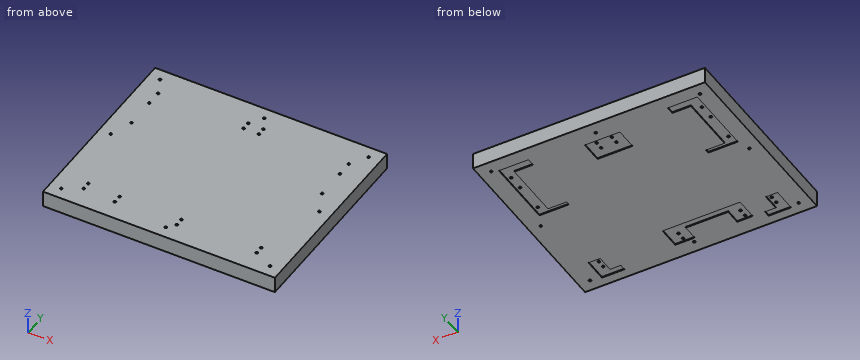
```python
from build123d import *

# Parameters (mm, degrees)
SKIZZE1_W                       = 300
SKIZZE1_H                       = 250
SKIZZE1_R                       = 1.6
AUFSATZ_LINEAR_AUSTRAGEN5_DEPTH = 21
SKIZZE2_R                       = 1.6
SKIZZE2_R_2                     = 1.5
SCHNITT_LINEAR_AUSTRAGEN2_DEPTH = 21
SKIZZE4_W                       = 45.307875895
SKIZZE4_H                       = 28.066825776
SCHNITT_LINEAR_AUSTRAGEN4_DEPTH = 1


with BuildPart() as part:
    # Skizze1 → Aufsatz-Linear austragen5 (new body)
    with BuildSketch(Plane.XY):
        with Locations((150, 125)):
            Rectangle(SKIZZE1_W, SKIZZE1_H)
        with Locations(Location((15, 15, 0), (0, 0, 180))):
            Circle(SKIZZE1_R, mode=Mode.SUBTRACT)
        with Locations(Location((285, 15, 0), (0, 0, 180))):
            Circle(SKIZZE1_R, mode=Mode.SUBTRACT)
        with Locations(Location((285, 235, 0), (0, 0, 180))):
            Circle(SKIZZE1_R, mode=Mode.SUBTRACT)
        with Locations(Location((15, 235, 0), (0, 0, 180))):
            Circle(SKIZZE1_R, mode=Mode.SUBTRACT)
        with Locations(Location((150, 15, 0), (0, 0, 180))):
            Circle(SKIZZE1_R, mode=Mode.SUBTRACT)
        with Locations(Location((285, 125, 0), (0, 0, 180))):
            Circle(SKIZZE1_R, mode=Mode.SUBTRACT)
        with Locations(Location((15, 125, 0), (0, 0, 180))):
            Circle(SKIZZE1_R, mode=Mode.SUBTRACT)
        with Locations(Location((150, 235, 0), (0, 0, 180))):
            Circle(SKIZZE1_R, mode=Mode.SUBTRACT)
    extrude(amount=AUFSATZ_LINEAR_AUSTRAGEN5_DEPTH)

    # Skizze2 → Schnitt-Linear austragen2 (cut)
    with BuildSketch(Plane.XY):
        with Locations(Location((158.603155074, 25.118294, 0), (0, 0, 180))):
            Circle(SKIZZE2_R)
        with Locations(Location((158.603155074, 35.36547744, 0), (0, 0, 180))):
            Circle(SKIZZE2_R)
        with Locations(Location((260.44562916, 27.513648646, 0), (0, 0, 180))):
            Circle(SKIZZE2_R)
        with Locations(Location((260.44562916, 37.512496181, 0), (0, 0, 180))):
            Circle(SKIZZE2_R)
        with Locations(Location((271.872836796, 153.81431076, 0), (0, 0, 180))):
            Circle(SKIZZE2_R)
        with Locations(Location((271.872850829, 193.508875377, 0), (0, 0, 180))):
            Circle(SKIZZE2_R)
        with Locations(Location((271.872850829, 213.356130747, 0), (0, 0, 180))):
            Circle(SKIZZE2_R)
        with Locations(Location((158.603451148, 218.134079373, 0), (0, 0, 180))):
            Circle(SKIZZE2_R)
        with Locations(Location((138.798289388, 208.167325209, 0), (0, 0, 180))):
            Circle(SKIZZE2_R)
        with Locations(Location((158.60315708, 208.111977885, 0), (0, 0, 180))):
            Circle(SKIZZE2_R)
        with Locations(Location((138.79828939, 218.357599581, 0), (0, 0, 180))):
            Circle(SKIZZE2_R)
        with Locations(Location((25.285732641, 193.508839291, 0), (0, 0, 180))):
            Circle(SKIZZE2_R)
        with Locations(Location((25.28570124, 213.065385973, 0), (0, 0, 180))):
            Circle(SKIZZE2_R)
        with Locations(Location((25.285701244, 153.814310759, 0), (0, 0, 180))):
            Circle(SKIZZE2_R)
        with Locations(Location((78.40440781, 25.118294004, 0), (0, 0, 180))):
            Circle(SKIZZE2_R)
        with Locations(Location((36.712941278, 27.513648641, 0), (0, 0, 180))):
            Circle(SKIZZE2_R_2)
        with Locations(Location((36.71294128, 37.560163652, 0), (0, 0, 180))):
            Circle(SKIZZE2_R)
        with Locations(Location((78.512463953, 35.365477438, 0), (0, 0, 180))):
            Circle(SKIZZE2_R)
    extrude(amount=SCHNITT_LINEAR_AUSTRAGEN2_DEPTH, mode=Mode.SUBTRACT)

    # Skizze4 → Schnitt-Linear austragen4 (cut)
    with BuildSketch(Plane.XY):
        Polygon((270.870452166, 12.477849124), (241.801240756, 12.477849124), (241.801240756, 20.496942202), (255.834654648, 20.496942202), (255.834654648, 42.549448169), (270.870452166, 42.549448169), align=None)
        Polygon((55.357331688, 12.477849124), (26.288120277, 12.477849124), (26.288120277, 42.549448169), (41.3239188, 42.549448169), (41.3239188, 20.496942202), (55.357331688, 20.496942202), align=None)
        Polygon((171.233227678, 20.99813552), (146.073322141, 20.99813552), (146.073322141, 41.045868217), (91.042295889, 41.045868217), (91.042295889, 20.99813552), (70.994563187, 20.99813552), (70.994563187, 49.064960293), (171.233227678, 49.064960293), align=None)
        with Locations((148.579289731, 208.444436236)):
            Rectangle(SKIZZE4_W, SKIZZE4_H)
        Polygon((276.884788012, 141.785725019), (238.794086862, 141.785725019), (238.794086862, 146.797660198), (262.851375124, 146.797660198), (262.851375124, 221.976656809), (238.794086862, 221.976656809), (238.794086862, 232.000523157), (276.884788012, 232.000523157), align=None)
        Polygon((58.364491591, 141.785725019), (20.273798467, 141.785725019), (20.273798467, 232.000523157), (58.364491591, 232.000523157), (58.364491591, 221.976656809), (34.307212355, 221.976656809), (34.307212355, 146.797660198), (58.364491591, 146.797660198), align=None)
    extrude(amount=SCHNITT_LINEAR_AUSTRAGEN4_DEPTH, mode=Mode.SUBTRACT)


solid = part.part
```
Part model, mm, in its own coordinate system. Round coordinates to 2 decimals unless told otherwise and drop trailing zeros. Write each loop counter-clockwise with the first axis right and the second up, starting at its lowest first coordinate (ties: lowest second). Pieces come first, ordered by that corner, then holes. Notation, with made-up numbers: M 41.5,29 L 88.5,29 A9 cw 88.5,36 Z; hole C 10,55.25 d2. An arc over 180 degrees is marked long. One line per question, with ' | ' between items.
(1) Probe line 1 along X through (y, z) = (125, 10.5); line 2 along Z through (x, y) = (33, 26). List the from-to ranges inside material, lowest first.
Answer key:
line 1: x = 0 to 13.4, 16.6 to 283.4, 286.6 to 300 | line 2: z = 1 to 21
(2) Saw through at A-A on x = 267. Write the cut outline in (y, z), then the cut area to 3 significant figures.
Answer key:
outline: M 0,0 L 12.48,0 L 12.48,1 L 42.55,1 L 42.55,0 L 141.79,0 L 141.79,1 L 232,1 L 232,0 L 250,0 L 250,21 L 0,21 Z | area: 5,130 mm^2
(3) Pin check, flat tips, straight feed: pin 1 (2.5 mm diameter, centred on x = 271.87, y = 153.81, fed in from -Z) (3 decimals); pin 2 (4 mm diameter, centred on x = 158.6, y = 208.11, fed in from -Z). Stop position of each tip, or through.
Answer key:
pin 1: passes through | pin 2: stops at z = 1
